Design review of the part built by this model. Coordinates are the model's own, in mm. Face numbers are marked on the shaded views. Give positions to 0.01 mm unless a question says otherwise; leave off trailing zeros. Order: outer loops, then holes, each group sorted by start corner. A loop starts at its lowest first (then second) coordinate and runs counter-clockwise, first axis right, second up. Notation, with made-up numbers: M 22,-3.75 L 65,-3.75 A27 cw 65,34.25 Z; hole C -14.5,-31.75 d11. An arc over 180 degrees is marked long. Answer as a JSON object with one key per item and string values.
from build123d import *

# Parameters (mm, degrees)
SKETCH1_R           = 9.5
SKETCH1_R_2         = 3.5
BOSS_EXTRUDE1_DEPTH = 13
FILLET1_R           = 4
SKETCH3_R           = 11
CUT_EXTRUDE1_DEPTH  = 2


with BuildPart() as part:
    # Sketch1 → Boss-Extrude1 (new body)
    with BuildSketch(Plane(origin=(0, 0, 0), x_dir=(1, 0, 0), z_dir=(0, 1, 0))):
        with BuildLine():
            Line((0.959404, 13.967087884), (29.596442563, 12))
            ThreePointArc((29.596442563, 12), (31, 0), (29.596442563, -12))
            Line((29.596442563, -12), (0.959404, -13.967087884))
            ThreePointArc((0.959404, -13.967087884), (-14, 0), (0.959404, 13.967087884))
        make_face()
        with Locations(Location((0, 0, 0), (0, 0, 90))):
            Circle(SKETCH1_R, mode=Mode.SUBTRACT)
        with Locations(Location((19, 0, 0), (0, 0, 90))):
            Circle(SKETCH1_R_2, mode=Mode.SUBTRACT)
    extrude(amount=BOSS_EXTRUDE1_DEPTH)

    # Fillet1
    fillet1_edges = [part.edges().sort_by_distance(p)[0] for p in [
        (29.596442563, 6.5, -12),
        (29.596442563, 6.5, 12),
    ]]
    fillet(fillet1_edges, radius=FILLET1_R)

    # Sketch3 → Cut-Extrude1 (cut)
    with BuildSketch(Plane(origin=(0, 13, 0), x_dir=(1, 0, 0), z_dir=(0, 1, 0))):
        with Locations(Location((0, 0, 0), (0, 0, 270))):
            Circle(SKETCH3_R)
    extrude(amount=-CUT_EXTRUDE1_DEPTH, mode=Mode.SUBTRACT)


solid = part.part
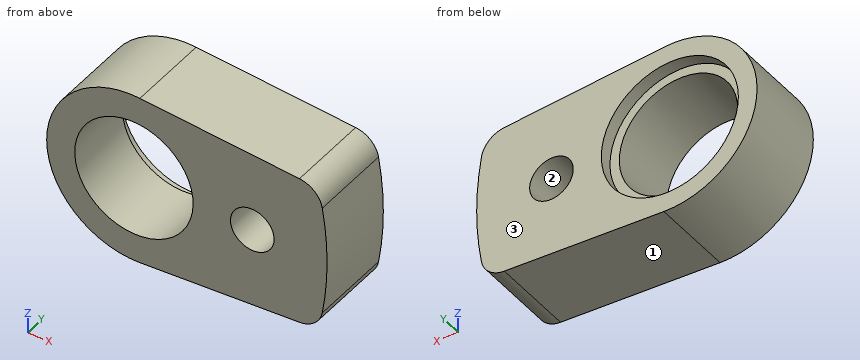
(1) To check wall thickness, follow L1, parallel to Z at x = 19, y = 9.5; L2, parallel to X at y = 9.5, z = -5.25; L3, parallel to Z at x = 4, y = 12. State the ranges of each line that lie inside material, in increasing order. Write a range as from..to.
Checked values:
{"L1": "z = -12.73..-3.5, 3.5..12.73", "L2": "x = -12.98..-7.92, 7.92..30.73", "L3": "z = -13.76..-10.25, 10.25..13.76"}
(2) Insertion check: pin 1 (6 mm diameter, centred on x = 7, y = 6, fed in from -Z); pin 2 (6 mm diameter, centred on y = 7.5, z = 3.5, fed in from +X); pin 3 (3 mm diameter, centred on y = 9.5, z = 7.5, fed in from -X). Each pin has a flat end and moves straight along its axis. Give the tip position at first contact, or say it passes through.
Checked values:
{"pin 1": "stops at z = -13.76", "pin 2": "stops at x = 31", "pin 3": "stops at x = -12.65"}
(3) Draft analysis for pull direction X (two halves, no side actions). For the marked faces 1, 2 and 3, state which applies: +X half, -X half, draft (parallel to the pull), parting line (faces both ways), or undercut.
Checked values:
{"face 1": "+X half", "face 2": "undercut", "face 3": "draft"}
(4) We need section A-A (z = 0). Write out the cut boundary in (x, y), plus the area to 3 significant figures.
Checked values:
{"outline": "M -14,0 L -9.5,0 L -9.5,11 L -11,11 L -11,13 L -14,13 Z; M 9.5,0 L 15.5,0 L 15.5,13 L 11,13 L 11,11 L 9.5,11 Z; M 22.5,0 L 31,0 L 31,13 L 22.5,13 Z", "area": "241 mm^2"}
(5) We need section C-C (x = 0). Write out the cut boundary in (y, z), plus the area to 3 significant figures.
Checked values:
{"outline": "M 0,-14 L 13,-14 L 13,-11 L 11,-11 L 11,-9.5 L 0,-9.5 Z; M 0,9.5 L 11,9.5 L 11,11 L 13,11 L 13,14 L 0,14 Z", "area": "111 mm^2"}
(6) We need section D-D (z = 7). Write out the cut boundary in (x, y), plus the area to 3 significant figures.
Checked values:
{"outline": "M -12.12,0 L -6.42,0 L -6.42,11 L -8.49,11 L -8.49,13 L -12.12,13 Z; M 6.42,0 L 30.53,0 L 30.53,13 L 8.49,13 L 8.49,11 L 6.42,11 Z", "area": "379 mm^2"}
(7) We need section B-B (y = 5.75). Write out the cut boundary in (x, z).
Checked values:
{"outline": "M 0.96,-13.97 L 26.57,-12.21 A4 ccw 30.23,-8.9 A52 ccw 30.23,8.9 A4 ccw 26.57,12.21 L 0.96,13.97 A14 ccw long Z; hole C 0,0 d19; hole C 19,0 d7"}
